Geometry check sheet. Reference: drawing and pictorial views, mm from the part's lowest x, y, z. Give positions to 0.01 mm unless a question says otherwise; leave off trailing zeros. Write each loop counter-clockwise with the first axis right and the second up, starting at its lowest first coordinate (ties: lowest second). Pieces come first, ordered by that corner, then holes. Notation, with made-up numbers: (-12.75, 87) - (-2.75, 87) arc R11 ccw to (-2.75, 101) - close; hole circle Ø5 at (30, -11.75). An arc over 180 degrees is marked (long way). Write item = value, one per line. Start each with the question number.
(1) Section check A-A, the plane z = 35. Enter the section's corners in (x, y), plus the area to 3 significant figures.
(2) Thickness scan on L1, parallel to X at y = 2.4, z = 60.5; L2, parallel to Z at x = 62, y = 0.95; L3, parallel to X at y = 2.35, z = 35. Record the ranges inside material, lowest first.
(3) Section check B-B, the plane x = 35. Enter the section's corners in (y, z).
(4) Depth check by flat-ended pin: pin 1 Ø1.5 at (y, z) = (1.5, 37.5) entering from -X. Enter the tip coordinate at first touch or a pass-through.
(5) Section check D-D, the plane x = 62. Enter the section's corners in (y, z).
(6) Section check C-C, the plane y = 1.95. Enter the section's corners in (x, z).
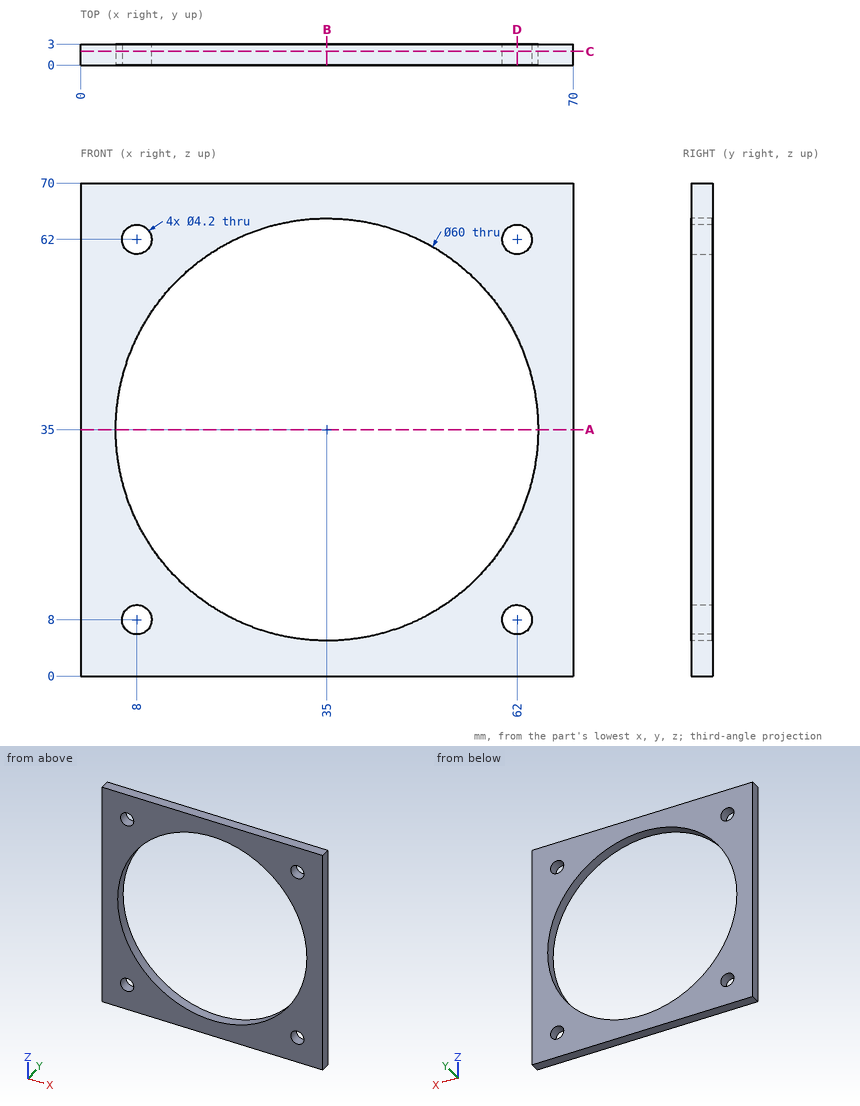
Model answer:
q1.outline = (0, 0) - (5, 0) - (5, 3) - (0, 3) - close; (65, 0) - (70, 0) - (70, 3) - (65, 3) - close
q1.area = 30.0 mm²
q2.L1 = 0 to 6.53, 9.47 to 19.2, 50.8 to 60.53, 63.47 to 70
q2.L2 = 0 to 5.9, 10.1 to 21.92, 48.08 to 59.9, 64.1 to 70
q2.L3 = 0 to 5, 65 to 70
q3.outline = (0, 0) - (3, 0) - (3, 5) - (0, 5) - close; (0, 65) - (3, 65) - (3, 70) - (0, 70) - close
q4.pin_1 = 0
q5.outline = (0, 0) - (3, 0) - (3, 5.9) - (0, 5.9) - close; (0, 10.1) - (3, 10.1) - (3, 21.92) - (0, 21.92) - close; (0, 48.08) - (3, 48.08) - (3, 59.9) - (0, 59.9) - close; (0, 64.1) - (3, 64.1) - (3, 70) - (0, 70) - close
q6.outline = (0, 0) - (70, 0) - (70, 70) - (0, 70) - close; hole circle Ø60 at (35, 35); hole circle Ø4.2 at (8, 8); hole circle Ø4.2 at (8, 62); hole circle Ø4.2 at (62, 8); hole circle Ø4.2 at (62, 62)
